Can you work these out from the model? Positions are in its coordinate system, mm. Coordinates: 2 decimals unless noted, no trailing zeros. Answer as a JSON object with one key per item and string values.
from build123d import *

# Parameters (mm, degrees)
SKETCH1_R           = 2.1
BOSS_EXTRUDE1_DEPTH = 800


with BuildPart() as part:
    # Sketch1 → Boss-Extrude1 (new body)
    with BuildSketch(Plane(origin=(0, 0, -600), x_dir=(-1, 0, 0), z_dir=(0, 0, -1))):
        with BuildLine():
            Line((10, -7), (10, 7))
            Line((10, 7), (8, 7))
            Line((8, 7), (8, 4))
            Line((8, 4), (7.060660172, 4))
            Line((7.060660172, 4), (4, 7.060660172))
            Line((4, 7.060660172), (4, 7.5))
            Line((4, 7.5), (3.750976592, 8.781114371))
            Line((3.750976592, 8.781114371), (3.933012702, 9.096410162))
            ThreePointArc((3.933012702, 9.096410162), (4, 9.346410162), (3.933012702, 9.596410162))
            Line((3.933012702, 9.596410162), (3.7, 10))
            Line((3.7, 10), (3.933012702, 10.403589838))
            ThreePointArc((3.933012702, 10.403589838), (3.982962913, 10.524180316), (4, 10.653589838))
            Line((4, 10.653589838), (4, 12.939339828))
            Line((4, 12.939339828), (7.060660172, 16))
            Line((7.060660172, 16), (8, 16))
            Line((8, 16), (8, 13))
            Line((8, 13), (10, 13))
            Line((10, 13), (10, 19))
            ThreePointArc((10, 19), (9.707106781, 19.707106781), (9, 20))
            Line((9, 20), (3, 20))
            Line((3, 20), (3, 18))
            Line((3, 18), (6, 18))
            Line((6, 18), (6, 17.060660172))
            Line((6, 17.060660172), (2.939339828, 14))
            Line((2.939339828, 14), (2.5, 14))
            Line((2.5, 14), (1.218885629, 13.750976592))
            Line((1.218885629, 13.750976592), (0.903589838, 13.933012702))
            ThreePointArc((0.903589838, 13.933012702), (0.653589838, 14), (0.403589838, 13.933012702))
            Line((0.403589838, 13.933012702), (0, 13.7))
            Line((0, 13.7), (-0.403589838, 13.933012702))
            ThreePointArc((-0.403589838, 13.933012702), (-0.524180316, 13.982962913), (-0.653589838, 14))
            Line((-0.653589838, 14), (-2.939339828, 14))
            Line((-2.939339828, 14), (-6, 17.060660172))
            Line((-6, 17.060660172), (-6, 18))
            Line((-6, 18), (-3, 18))
            Line((-3, 18), (-3, 20))
            Line((-3, 20), (-9, 20))
            ThreePointArc((-9, 20), (-9.707106781, 19.707106781), (-10, 19))
            Line((-10, 19), (-10, 13))
            Line((-10, 13), (-8, 13))
            Line((-8, 13), (-8, 16))
            Line((-8, 16), (-7.060660172, 16))
            Line((-7.060660172, 16), (-4, 12.939339828))
            Line((-4, 12.939339828), (-4, 12.5))
            Line((-4, 12.5), (-3.750976592, 11.218885629))
            Line((-3.750976592, 11.218885629), (-3.933012702, 10.903589838))
            ThreePointArc((-3.933012702, 10.903589838), (-4, 10.653589838), (-3.933012702, 10.403589838))
            Line((-3.933012702, 10.403589838), (-3.7, 10))
            Line((-3.7, 10), (-3.933012702, 9.596410162))
            ThreePointArc((-3.933012702, 9.596410162), (-3.982962913, 9.475819684), (-4, 9.346410162))
            Line((-4, 9.346410162), (-4, 7.060660172))
            Line((-4, 7.060660172), (-7.060660172, 4))
            Line((-7.060660172, 4), (-8, 4))
            Line((-8, 4), (-8, 7))
            Line((-8, 7), (-10, 7))
            Line((-10, 7), (-10, -7))
            Line((-10, -7), (-8, -7))
            Line((-8, -7), (-8, -4))
            Line((-8, -4), (-7.060660172, -4))
            Line((-7.060660172, -4), (-4, -7.060660172))
            Line((-4, -7.060660172), (-4, -9.346410162))
            ThreePointArc((-4, -9.346410162), (-3.982962913, -9.475819684), (-3.933012702, -9.596410162))
            Line((-3.933012702, -9.596410162), (-3.7, -10))
            Line((-3.7, -10), (-3.933012702, -10.403589838))
            ThreePointArc((-3.933012702, -10.403589838), (-4, -10.653589838), (-3.933012702, -10.903589838))
            Line((-3.933012702, -10.903589838), (-3.750976592, -11.218885629))
            Line((-3.750976592, -11.218885629), (-4, -12.5))
            Line((-4, -12.5), (-4, -12.939339828))
            Line((-4, -12.939339828), (-7.060660172, -16))
            Line((-7.060660172, -16), (-8, -16))
            Line((-8, -16), (-8, -13))
            Line((-8, -13), (-10, -13))
            Line((-10, -13), (-10, -19))
            ThreePointArc((-10, -19), (-9.707106781, -19.707106781), (-9, -20))
            Line((-9, -20), (-3, -20))
            Line((-3, -20), (-3, -18))
            Line((-3, -18), (-6, -18))
            Line((-6, -18), (-6, -17.060660172))
            Line((-6, -17.060660172), (-2.939339828, -14))
            Line((-2.939339828, -14), (-0.653589838, -14))
            ThreePointArc((-0.653589838, -14), (-0.524180316, -13.982962913), (-0.403589838, -13.933012702))
            Line((-0.403589838, -13.933012702), (0, -13.7))
            Line((0, -13.7), (0.403589839, -13.933012702))
            ThreePointArc((0.403589839, -13.933012702), (0.653589839, -14), (0.903589838, -13.933012702))
            Line((0.903589838, -13.933012702), (1.218885629, -13.750976592))
            Line((1.218885629, -13.750976592), (2.5, -14))
            Line((2.5, -14), (2.939339828, -14))
            Line((2.939339828, -14), (6, -17.060660172))
            Line((6, -17.060660172), (6, -18))
            Line((6, -18), (3, -18))
            Line((3, -18), (3, -20))
            Line((3, -20), (9, -20))
            ThreePointArc((9, -20), (9.707106781, -19.707106781), (10, -19))
            Line((10, -19), (10, -13))
            Line((10, -13), (8, -13))
            Line((8, -13), (8, -16))
            Line((8, -16), (7.060660172, -16))
            Line((7.060660172, -16), (4, -12.939339828))
            Line((4, -12.939339828), (4, -10.653589838))
            ThreePointArc((4, -10.653589838), (3.982962913, -10.524180316), (3.933012702, -10.403589838))
            Line((3.933012702, -10.403589838), (3.7, -10))
            Line((3.7, -10), (3.933012702, -9.596410162))
            ThreePointArc((3.933012702, -9.596410162), (4, -9.346410162), (3.933012702, -9.096410162))
            Line((3.933012702, -9.096410162), (3.750976592, -8.781114371))
            Line((3.750976592, -8.781114371), (4, -7.5))
            Line((4, -7.5), (4, -7.060660172))
            Line((4, -7.060660172), (7.060660172, -4))
            Line((7.060660172, -4), (8, -4))
            Line((8, -4), (8, -7))
            Line((8, -7), (10, -7))
        make_face()
        with Locations((0, -10)):
            Circle(SKETCH1_R, mode=Mode.SUBTRACT)
        with Locations((0, 10)):
            Circle(SKETCH1_R, mode=Mode.SUBTRACT)
        with BuildLine():
            Line((8, 1.7), (8, -1.7))
            ThreePointArc((8, -1.7), (7.912132034, -1.912132034), (7.7, -2))
            Line((7.7, -2), (7.063603897, -2))
            ThreePointArc((7.063603897, -2), (6.948798867, -2.02283614), (6.851471863, -2.087867966))
            Line((6.851471863, -2.087867966), (2.939339828, -6))
            Line((2.939339828, -6), (-2.939339828, -6))
            Line((-2.939339828, -6), (-6.851471863, -2.087867966))
            ThreePointArc((-6.851471863, -2.087867966), (-6.948798867, -2.02283614), (-7.063603897, -2))
            Line((-7.063603897, -2), (-7.7, -2))
            ThreePointArc((-7.7, -2), (-7.912132034, -1.912132034), (-8, -1.7))
            Line((-8, -1.7), (-8, 1.7))
            ThreePointArc((-8, 1.7), (-7.912132034, 1.912132034), (-7.7, 2))
            Line((-7.7, 2), (-7.063603897, 2))
            ThreePointArc((-7.063603897, 2), (-6.948798867, 2.02283614), (-6.851471863, 2.087867966))
            Line((-6.851471863, 2.087867966), (-2.939339828, 6))
            Line((-2.939339828, 6), (2.939339828, 6))
            Line((2.939339828, 6), (6.851471863, 2.087867966))
            ThreePointArc((6.851471863, 2.087867966), (6.948798867, 2.02283614), (7.063603897, 2))
            Line((7.063603897, 2), (7.7, 2))
            ThreePointArc((7.7, 2), (7.912132034, 1.912132034), (8, 1.7))
        make_face(mode=Mode.SUBTRACT)
    extrude(amount=-BOSS_EXTRUDE1_DEPTH)


solid = part.part
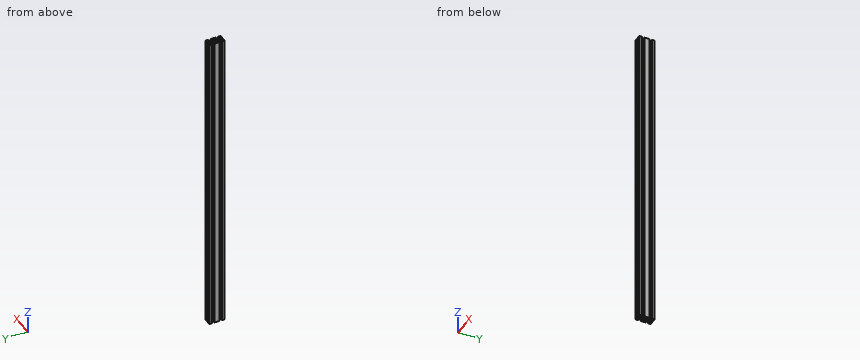
Item 1: Please list where these lines run through material, in increasing order: line 1 (Y direction, x = 0, z = 19); line 2 (Y direction, x = -0.75, z = -139); line 3 (Y direction, x = 2.25, z = -511.5).
Answers follow:
{"line 1": "y = -13.7 to -12.1, -7.9 to -6, 6 to 7.9, 12.1 to 13.7", "line 2": "y = -13.99 to -11.96, -8.04 to -6, 6 to 8.04, 11.96 to 13.99", "line 3": "y = -14 to -6, 6 to 14"}
Item 2: I'm going to push flat-ended pins straight in: pin 1 (1.5 mm diameter, centred on x = -2, z = -180, fed in from +Y); pin 2 (2.5 mm diameter, centred on x = 0, y = -10, fed in from +Z); pin 3 (3 mm diameter, centred on x = 7.5, y = -12, fed in from +Z); pin 4 (0.5 mm diameter, centred on x = -2.5, z = -219.5, fed in from -Y). Where does each tip first touch, or does it pass through?
Answers follow:
{"pin 1": "stops at y = 14", "pin 2": "passes through", "pin 3": "stops at z = 200", "pin 4": "stops at y = -14"}
Item 3: I want a section at A-A, the plane z = 150.5. Give the number of separate pieces and of enclosed holes in the cut face, plus the area to 3 significant figures.
Answers follow:
{"separate pieces": "1", "enclosed holes": "3", "area": "322 mm^2"}
